Autodesk Fusion 360 part; units mm, degrees
sketch "Sketch1" plane through (0, 0, 0) normal (0, 1, 0) x (1, 0, 0)
  line L0 (110, 0) -> (41.4831, 0)
  line L1 (51.9615, -45) -> (110, -45)
  line L2 (110, -45) -> (110, 0)
  line L3 (41.4831, 0) -> (0, 0)
  line L4 (0, 0) -> (51.9615, -45)
  dimension "d1" = 110
  dimension "d2" = 45
  dimension "d4" = 58.0385
extrude "Extrude1" add sketch "Sketch1" along normal blind 5
sketch "Sketch2" plane through (0, 0, 0) normal (0, -1, 0) x (1, 0, 0)
  line L0 (51.9615, 45) -> (0, 0)
  line L1 (0, 0) -> (110, 0)
  line L2 (110, 0) -> (110, 45)
  line L3 (110, 45) -> (51.9615, 45)
  line L4 (55, 0) -> (85, 0)
  line L5 (85, 0) -> (85, 30)
  line L6 (85, 30) -> (55, 30)
  line L7 (55, 30) -> (55, 0)
  line L8 (44.1386, 5) -> (48.1184, 11.8931)
  line L9 (48.1184, 11.8931) -> (44.1386, 18.7862)
  line L10 (44.1386, 18.7862) -> (36.1791, 18.7862)
  line L11 (36.1791, 18.7862) -> (32.1994, 11.8931)
  line L12 (32.1994, 11.8931) -> (36.1791, 5)
  line L13 (36.1791, 5) -> (44.1386, 5)
  point P0 (40.1589, 11.8931)
  dimension "d8" = 25
  dimension "d9" = 15
  dimension "d11" = 5
extrude "Extrude2" cut sketch "Sketch2" against normal through all contours L1 L4 L5 L6 L7
extrude "Extrude3" cut sketch "Sketch2" against normal through all contours L8 L9 L10 L11 L12 L13
Here's how the part is built. I have some questions about the finished solid (model axes, mm). A direction names the side the tool comes from. Coordinates: 2 decimals unless noted, no trailing zeros. Order: outer loops, then holes, each group sorted by start corner. A loop starts at its lowest first (then second) coordinate and runs counter-clockwise, first axis right, second up. Notation, with made-up numbers: (14, 18) - (60, 18) arc R31 ccw to (60, 55) - close; hole circle Ø5 at (2.5, -39.75). An arc over 180 degrees is marked (long way). One line per question, with ' | ' between items.
(1) Suppose I cut it at C-C on x = 46. List the corners of the cut face in (y, z) for me.
Report:
outline: (0, 0) - (5, 0) - (5, 8.22) - (0, 8.22) - close; (0, 15.56) - (5, 15.56) - (5, 39.84) - (0, 39.84) - close
(2) If we mould it in two halves opening along Z, with no side actions, what happens to faces 1 (the flat face through (98, 2, 0)), 2 (the flat face through (34.22, 2.46, 15.39)), 3 (the flat face through (81, 2, 45))? For each: pulls with the +Z half, pulls with the -Z half, needs draft (parallel to the pull), parting line crosses it, or undercut.
Report:
face 1: pulls with the -Z half | face 2: undercut | face 3: pulls with the +Z half
(3) For faces 4 (the flat face through (46.156, 2.465, 15.291)), 5 (the flat face through (85, 2, 15)), 6 (the flat face through (110, 2, 23)), which set-ups out of +Z, -Z, +X, -X, +Y, -Y let a thin tool reach every point of the face, with its end or its side?
Report:
face 4: +Y, -Y | face 5: -Z, +Y, -Y | face 6: +Z, -Z, +X, +Y, -Y
(4) Will these pins go through, and if not, where does the flat tip stop? pin 1 (2.5 mm diameter, centred on x = 68.5, y = 3.5, fed in from -Z); pin 2 (1.5 mm diameter, centred on x = 39, y = 3.5, fed in from +Z).
Report:
pin 1: stops at z = 30 | pin 2: stops at z = 34.42
(5) Suppose I cut it at B-B on z = 15.5. List the corners of the cut face in (x, y) for me.
Report:
outline: (17.9, 0) - (34.28, 0) - (34.28, 5) - (17.9, 5) - close; (46.04, 0) - (55, 0) - (55, 5) - (46.04, 5) - close; (85, 0) - (110, 0) - (110, 5) - (85, 5) - close
(6) If I drill on L1, parallel to Z at x = 72.5, y = 2.45; L2, parallel to X at y = 1.4, z = 16.5; L3, parallel to Z at x = 45.5, y = 2.85, over which ranges is the centre line in solid material (lowest first)?
Report:
L1: z = 30 to 45 | L2: x = 19.05 to 34.86, 45.46 to 55, 85 to 110 | L3: z = 0 to 7.36, 16.43 to 39.4
(7) Suppose I cut it at D-D on z = 28. List the corners of the cut face in (x, y) for me.
Report:
outline: (32.33, 0) - (55, 0) - (55, 5) - (32.33, 5) - close; (85, 0) - (110, 0) - (110, 5) - (85, 5) - close
(8) Suppose I cut it at A-A on y = 1.7. List the corners of the cut face in (x, z) for me, and give its area (3 significant figures).
Report:
outline: (0, 0) - (55, 0) - (55, 30) - (85, 30) - (85, 0) - (110, 0) - (110, 45) - (51.96, 45) - close; hole (32.2, 11.89) - (36.18, 5) - (44.14, 5) - (48.12, 11.89) - (44.14, 18.79) - (36.18, 18.79) - close | area: 2,720 mm2
